Model file for the job. Use its own axes, mm. A direction names the side the tool comes from. Round coordinates to 2 decimals unless told otherwise and drop trailing zeros. Order: outer loops, then holes, each group sorted by start corner. A loop starts at its lowest first (then second) coordinate and runs counter-clockwise, first axis right, second up. Notation, with made-up numbers: (8.25, 85) - (52.25, 85) arc R22 cw to (52.25, 123) - close; hole circle Ø2 at (3, 88.5). An arc over 180 degrees is marked (long way). Write item = value, one per line.
```python
from build123d import *

# Parameters (mm, degrees)
SKETCH2_W              = 191.135
SKETCH2_H              = 23.622
MOUNT_BAR_DEPTH        = 6.35
MOUNT_FEATURE_DEPTH    = 12.7
FILLET1_R              = 2.54
SKETCH5_R              = 1.397
MOUNT_HOLES_DEPTH      = 10.795
SKETCH6_W              = 53.34
SKETCH6_H              = 6.985
BOSS_EXTRUDE5_DEPTH    = 12.7
FILLET2_R              = 2.54
CHAMFER1_SIZE          = 2.54
CHAMFER2_SIZE          = 2.159
SKETCH7_W              = 165.735
SKETCH7_H              = 8.382
WEIGHT_REDUCTION_DEPTH = 104.551367988
FILLET3_R              = 2.54


with BuildPart() as part:
    # Sketch2 → Mount-Bar (new, symmetric)
    with BuildSketch(Plane(origin=(0, 0, 0), x_dir=(1, 0, 0), z_dir=(0, 1, 0))):
        Rectangle(SKETCH2_W, SKETCH2_H)
    extrude(amount=MOUNT_BAR_DEPTH, both=True)

    # Sketch4 → Mount-Feature (add)
    with BuildSketch(Plane(origin=(0, 6.35, 0), x_dir=(1, 0, 0), z_dir=(0, 1, 0))):
        Polygon((-31.75, 11.811), (-31.75, 26.289), (31.75, 26.289), (31.75, 11.811), (36.195, 11.811), (36.195, 30.734), (-36.195, 30.734), (-36.195, 11.811), align=None)
    extrude(amount=-MOUNT_FEATURE_DEPTH)

    # Fillet1
    fillet1_edges = [part.edges().sort_by_distance(p)[0] for p in [
        (-31.75, 0, -11.811),
        (-36.195, 0, -11.811),
        (36.195, 0, -11.811),
        (31.75, 0, -11.811),
        (31.75, 0, -26.289),
        (-31.75, 0, -26.289),
    ]]
    fillet(fillet1_edges, radius=FILLET1_R)

    # Sketch5 → Mount-Holes (cut)
    with BuildSketch(Plane.ZY.offset(95.5675)):
        with Locations((-4.028538113, 1.878538173)):
            Circle(SKETCH5_R)
        with Locations((4.028538113, -1.878538173)):
            Circle(SKETCH5_R)
    mount_holes = extrude(amount=-MOUNT_HOLES_DEPTH, mode=Mode.SUBTRACT)

    # Mirror1: Mount-Holes across plane
    add(mount_holes.mirror(Plane(origin=(0, 0, 0), x_dir=(0, 0, 1), z_dir=(1, 0, 0))), mode=Mode.SUBTRACT)

    # Sketch6 → Boss-Extrude5 (add)
    with BuildSketch(Plane.XZ.offset(6.35)):
        with Locations((0, -8.3185)):
            Rectangle(SKETCH6_W, SKETCH6_H)
    extrude(amount=BOSS_EXTRUDE5_DEPTH)

    # Fillet2
    fillet2_edges = [part.edges().sort_by_distance(p)[0] for p in [
        (-26.67, -6.35, -8.3185),
        (0, -6.35, -4.826),
        (26.67, -6.35, -8.3185),
    ]]
    fillet(fillet2_edges, radius=FILLET2_R)

    # Chamfer1
    chamfer1_edges = [part.edges().sort_by_distance(p)[0] for p in [
        (0, -19.05, -4.826),
        (-36.195, 0, -30.734),
        (36.195, 0, -30.734),
    ]]
    chamfer(chamfer1_edges, length=CHAMFER1_SIZE)

    # Chamfer2
    chamfer2_edges = [part.edges().sort_by_distance(p)[0] for p in [
        (-95.5675, 0, -11.811),
        (95.5675, 0, -11.811),
        (95.5675, 0, 11.811),
        (-95.5675, 0, 11.811),
    ]]
    chamfer(chamfer2_edges, length=CHAMFER2_SIZE)

    # Sketch7 → weight-reduction (cut, through all)
    with BuildSketch(Plane(origin=(0, 6.35, 0), x_dir=(1, 0, 0), z_dir=(0, 1, 0))):
        Rectangle(SKETCH7_W, SKETCH7_H)
    extrude(amount=-WEIGHT_REDUCTION_DEPTH, mode=Mode.SUBTRACT)

    # Fillet3
    fillet3_edges = [part.edges().sort_by_distance(p)[0] for p in [
        (-82.8675, 0, 4.191),
        (82.8675, 0, -4.191),
        (82.8675, 0, 4.191),
        (-82.8675, 0, -4.191),
    ]]
    fillet(fillet3_edges, radius=FILLET3_R)


solid = part.part
```
1) Wall check: line 1 along Z through (x, y) = (71, 2.5); line 2 along X through (y, z) = (0, -1); line 3 along X through (y, z) = (-5.5, -18) (3 decimals). Give the ranges that are in metal, low to high.
Conclusion:
line_1 = -11.81 to -4.19, 4.19 to 11.81
line_2 = -95.57 to -82.87, 82.87 to 95.57
line_3 = -36.195 to -31.75, 31.75 to 36.195
2) Flat gauge pins, fed straight in: pin 1 Ø3 at (y, z) = (2.5, -17.5) entering from +X (3 decimals); pin 2 Ø6.5 at (x, y) = (59, -2) entering from -Z; pin 3 Ø1.4 at (y, z) = (2, -4) entering from -X. Where does each tip first touch, or does it go through?
Conclusion:
pin_1 = 36.195
pin_2 = -11.81
pin_3 = -84.77
3) Cut at A-A (z = -16). Write the cut outline in (x, y) (3 decimals).
Conclusion:
outline = (-36.195, -6.35) - (-31.75, -6.35) - (-31.75, 6.35) - (-36.195, 6.35) - close; (31.75, -6.35) - (36.195, -6.35) - (36.195, 6.35) - (31.75, 6.35) - close
4) Cut at C-C (x = -68). Write the cut outline in (y, z).
Conclusion:
outline = (-6.35, -11.81) - (6.35, -11.81) - (6.35, -4.19) - (-6.35, -4.19) - close; (-6.35, 4.19) - (6.35, 4.19) - (6.35, 11.81) - (-6.35, 11.81) - close
5) Cut at B-B (x = -1). Write the cut outline in (y, z).
Conclusion:
outline = (-19.05, -11.81) - (6.35, -11.81) - (6.35, -4.19) - (-7.21, -4.19) arc R2.54 cw to (-8.89, -4.83) - (-16.51, -4.83) - (-19.05, -7.37) - close; (-6.35, -30.73) - (6.35, -30.73) - (6.35, -26.29) - (-6.35, -26.29) - close; (-6.35, 4.19) - (6.35, 4.19) - (6.35, 11.81) - (-6.35, 11.81) - close
6) Mould opens along X. For faces 1 (the face through (-36.195, 0, -21)), 2 (the face through (36.195, 0, -21)), 3 (the face through (0, 0, -26.289)) say: +X half, -X half, draft (parallel to the pull), parting line (faces both ways), or undercut.
Conclusion:
face_1 = -X half
face_2 = +X half
face_3 = undercut
7) Cut at D-D (y = -13.25). Write the cut outline in (x, z), and give its area (3 significant figures).
Conclusion:
outline = (-26.67, -11.81) - (26.67, -11.81) - (26.67, -4.83) - (-26.67, -4.83) - close
area = 373 mm^2
8) 3-axis set-ups, long thin cutter, end or side, ignore diameter. For faces 4 (the face through (-66, 0, -11.811)), 5 (the face through (-26.67, -14, -8)), 6 (the face through (0, -6, -11.811)), 7 (the face through (0, -13, -4.826)): which of +Z, -Z, +X, -X, +Y, -Y reach the whole face in a straight line?
Conclusion:
face_4 = -Z, -X, +Y, -Y
face_5 = +Z, -Z, -X, -Y
face_6 = +Y, -Y
face_7 = +Z, +X, -X, -Y
